```python
from build123d import *

# Parameters (mm, degrees)
SKETCH2_W                = 2
SKETCH2_H                = 162.039928857
SKETCH5_W                = 72.783621468
SKETCH5_H                = 192.84631039
CUT_EXTRUDE1_DEPTH       = 94.869329042
BOSS_EXTRUDE1_REACH      = 97.869
BOSS_EXTRUDE1_END_RADIUS = 14
BOSS_EXTRUDE1_START      = -2
SKETCH4_W                = 15.457813272
SKETCH4_H                = 5
SKETCH4_W_2              = 16.763190872
SKETCH4_H_2              = 4
SKETCH4_W_3              = 1.5
SKETCH4_H_3              = 48.554461885
BOSS_EXTRUDE2_REACH      = 105.369
BOSS_EXTRUDE2_START      = -9.5
SKETCH4_4_W              = 8
SKETCH4_4_H              = 48.554461885
SKETCH6_R                = 2
CUT_EXTRUDE2_DEPTH       = 4


with BuildPart() as part:
    # Sketch1 → Revolve1 (revolve)
    with BuildSketch(Plane.XY, mode=Mode.PRIVATE) as revolve1_sk:
        with BuildLine():
            Line((6.354000149, 87.279039692), (16, 71))
            Line((16, 71), (0, 71))
            Line((0, 71), (0, 91))
            add(Edge.make_bspline(
                [(0, 91), (4.668589185, 91.723642341), (6.354000149, 87.279039692)],
                knots=[0, 0, 0, 1, 1, 1], degree=2))
        make_face()
    revolve(revolve1_sk.sketch.rotate(Axis((0, 91, 0), (0, -1, 0)), 180), axis=Axis((0, 91, 0), (0, -1, 0)))

    # Sketch2 → Revolve2 (revolve)
    with BuildSketch(Plane.XY, mode=Mode.PRIVATE) as revolve2_sk:
        with Locations((15, -10.019964429)):
            Rectangle(SKETCH2_W, SKETCH2_H)
    revolve(revolve2_sk.sketch.rotate(Axis((0, 91, 0), (0, -1, 0)), 180), axis=Axis((0, 91, 0), (0, -1, 0)))

    # Sketch5 → Cut-Extrude1 (cut, through all)
    with BuildSketch(Plane.XY):
        Rectangle(SKETCH5_W, SKETCH5_H)
    extrude(amount=CUT_EXTRUDE1_DEPTH, mode=Mode.SUBTRACT)

    # Boss-Extrude1: up to this cylinder (the profile starts inside it)
    boss_extrude1_end = Plane(origin=(0, 0.172402, 0), z_dir=(0, 1, 0)) * Cylinder(BOSS_EXTRUDE1_END_RADIUS, 313.082804, mode=Mode.PRIVATE)
    # Sketch4 → Boss-Extrude1 (add, up to the surface)
    with BuildSketch(Plane.XY.offset(BOSS_EXTRUDE1_START), mode=Mode.PRIVATE) as boss_extrude1_sk1:
        with Locations((0, 13.5)):
            Rectangle(SKETCH4_W, SKETCH4_H)
    boss_extrude1_tool1 = extrude(boss_extrude1_sk1.sketch, amount=-BOSS_EXTRUDE1_REACH, mode=Mode.PRIVATE) & boss_extrude1_end
    add(boss_extrude1_tool1.solids().sort_by_distance((0, 13.5, -2))[0])
    # Sketch4 → Boss-Extrude1 (add, up to the surface)
    with BuildSketch(Plane.XY.offset(BOSS_EXTRUDE1_START), mode=Mode.PRIVATE) as boss_extrude1_sk2:
        with Locations((0, -44)):
            Rectangle(SKETCH4_W_2, SKETCH4_H_2)
    boss_extrude1_tool2 = extrude(boss_extrude1_sk2.sketch, amount=-BOSS_EXTRUDE1_REACH, mode=Mode.PRIVATE) & boss_extrude1_end
    add(boss_extrude1_tool2.solids().sort_by_distance((0, -44, -2))[0])
    # Sketch4 → Boss-Extrude1 (add, up to the surface)
    with BuildSketch(Plane.XY.offset(BOSS_EXTRUDE1_START), mode=Mode.PRIVATE) as boss_extrude1_sk3:
        with Locations((4.75, 44.344804049)):
            Rectangle(SKETCH4_W_3, SKETCH4_H_3)
    boss_extrude1_tool3 = extrude(boss_extrude1_sk3.sketch, amount=-BOSS_EXTRUDE1_REACH, mode=Mode.PRIVATE) & boss_extrude1_end
    add(boss_extrude1_tool3.solids().sort_by_distance((4.75, 44.344804, -2))[0])
    # Sketch4 → Boss-Extrude1 (add, up to the surface)
    with BuildSketch(Plane.XY.offset(BOSS_EXTRUDE1_START), mode=Mode.PRIVATE) as boss_extrude1_sk4:
        with Locations((-4.75, 44.344804049)):
            Rectangle(SKETCH4_W_3, SKETCH4_H_3)
    boss_extrude1_tool4 = extrude(boss_extrude1_sk4.sketch, amount=-BOSS_EXTRUDE1_REACH, mode=Mode.PRIVATE) & boss_extrude1_end
    add(boss_extrude1_tool4.solids().sort_by_distance((-4.75, 44.344804, -2))[0])

    # Sketch4<4> → Boss-Extrude2 (add, up to next)
    with BuildSketch(Plane.XY.offset(BOSS_EXTRUDE2_START), mode=Mode.PRIVATE) as boss_extrude2_sk1:
        with Locations((0, 44.344804049)):
            Rectangle(SKETCH4_4_W, SKETCH4_4_H)
    boss_extrude2_tool1 = extrude(boss_extrude2_sk1.sketch, amount=-BOSS_EXTRUDE2_REACH, mode=Mode.PRIVATE) - part.part
    add(boss_extrude2_tool1.solids().sort_by_distance((0, 44.344804, -9.5))[0])

    # Sketch6 → Cut-Extrude2 (cut)
    with BuildSketch(Plane.XY):
        with Locations((4.579301858, 78.367512537)):
            Circle(SKETCH6_R)
        with Locations((-3.558513385, 76.255407818)):
            Circle(SKETCH6_R)
        with Locations((-0.919296183, 85.076551058)):
            Circle(SKETCH6_R)
    extrude(amount=-CUT_EXTRUDE2_DEPTH, mode=Mode.SUBTRACT)


solid = part.part
```
Model file for the job. Use its own axes, mm. A direction names the side the tool comes from. Round coordinates to 2 decimals unless told otherwise and drop trailing zeros. Loops run counter-clockwise (first coordinate to the right, second up) from the corner with the lowest first, then second, coordinate; pieces in that order, holes last. Notation, with made-up numbers: M 78.5,-38.5 L 106.5,-38.5 A18 ccw 106.5,-22.5 Z; hole C 27.5,-5 d5. An arc over 180 degrees is marked long. Put each result on its own line as item: value. Start each with the question number.
Item 1: Drill centre lines: line 1 along Y through (x, z) = (5, -4.75); line 2 along X through (y, z) = (31.5, -12.75); line 3 along X through (y, z) = (22, -8). Where is each one in solid material? Low to high.
Item 2: Drop flat-ended pins along their axis: P1, Ø4, axis at x = 4.5, z = -9.5, coming from the -Y side; P2, Ø2, axis at y = 71.5, z = -7.5, coming from the +X side; P3, Ø1.5, axis at x = -6, y = -27.5, coming from the +Z side. Give the stop position or say it passes through.
Item 3: 3-axis set-ups, long thin cutter, end or side, ignore diameter. For faces 4 (the face through (0, 45, -9.5)), 5 (the face through (0, -44, -2)): which of +Z, -Z, +X, -X, +Y, -Y reach the whole face in a straight line?
Item 4: Mould opens along X. For faces 1 (the face through (-0.224, 80.834, -10.17)), 2 (the face through (0, 68.622, -11)), 3 (the face through (2.3, -91.04, -14)) say: released by +X, released by -X, zero draft, split by the parting line, or undercut.
Item 5: Cut at A-A (y = -32). List the corners of the cut face in (x, z), then the cut area to 3 significant figures.
Answer block:
1. line 1: -46 to -42, 11 to 16, 20.07 to 68.62, 71 to 86.36
1. line 2: -9.67 to -5.78, -5.5 to 5.5, 5.78 to 9.67
1. line 3: -13.86 to -11.49, -5.5 to -4, 4 to 5.5, 11.49 to 13.86
2. P1: y = -46
2. P2: x = 14.56
2. P3: z = -12.27
3. face 4: +Z
3. face 5: +Z, -Y
4. face 1: split by the parting line
4. face 2: undercut
4. face 3: zero draft
5. outline: M -16,0 A16 ccw 16,0 L 14,0 A14 cw -14,0 Z
5. area: 94.2 mm2
